```python
from build123d import *

# Parameters (mm, degrees)
SKETCH1_W               = 40
SKETCH1_H               = 60
BOSS_EXTRUDE4_DEPTH     = 2
FILLET1_R               = 5
SKETCH12_R              = 1
CUT_EXTRUDE6_DEPTH      = 12
CUT_EXTRUDE7_DEPTH      = 8
CUT_EXTRUDE7_DEPTH_BACK = 10
SKETCH13_R              = 1


with BuildPart() as part:
    # Sketch1 → Boss-Extrude4 (new body)
    with BuildSketch(Plane.XY):
        with Locations((-45.9850693, -3.193565597)):
            Rectangle(SKETCH1_W, SKETCH1_H)
    extrude(amount=-BOSS_EXTRUDE4_DEPTH)

    # Fillet1
    fillet1_edges = [part.edges().sort_by_distance(p)[0] for p in [
        (-65.9850693, 26.806434403, -1),
        (-65.9850693, -33.193565597, -1),
        (-25.9850693, -33.193565597, -1),
        (-25.9850693, 26.806434403, -1),
    ]]
    fillet(fillet1_edges, radius=FILLET1_R)

    # Sketch12 → Cut-Extrude6 (cut)
    with BuildSketch(Plane(origin=(0, 0, -2), x_dir=(-1, 0, 0), z_dir=(0, 0, -1))):
        with Locations((45.9850693, -3.193565597)):
            Circle(SKETCH12_R)
    extrude(amount=-CUT_EXTRUDE6_DEPTH, mode=Mode.SUBTRACT)

    # Sketch13 → Cut-Extrude7 (cut, two sides: drawn at the far end of the back side and taken through both)
    with BuildSketch(Plane(origin=(0, 0, -2), x_dir=(-1, 0, 0), z_dir=(0, 0, -1)).offset(-CUT_EXTRUDE7_DEPTH_BACK)):
        with Locations((55.9850693, 4.306434403)):
            Circle(SKETCH13_R)
        with Locations((55.9850693, -10.693565597)):
            Circle(SKETCH13_R)
    extrude(amount=CUT_EXTRUDE7_DEPTH + CUT_EXTRUDE7_DEPTH_BACK, mode=Mode.SUBTRACT)


solid = part.part
```
The model under review builds one solid part; all positions refer to its coordinate system, in mm. Round coordinates to 2 decimals unless told otherwise and drop trailing zeros. Loops run counter-clockwise (first coordinate to the right, second up) from the corner with the lowest first, then second, coordinate; pieces in that order, holes last. Notation, with made-up numbers: M 53,-16.75 L 68,-16.75 A27 ccw 68,14.25 Z; hole C 20,48.5 d7. An arc over 180 degrees is marked long. Put each result on its own line as item: value.
Q1. For pin 1 (1.2 mm diameter, centred on x = -45.99, y = -3.19, fed in from -Z), flat-tipped, find the tip position at first contact; note if it passes through.
Result set:
pin 1: passes through
Q2. Mouldability with a two-part tool opening along Y and no side actions: class faces 1 (the cylindrical face through (-56.939, -10.393, -0.986)), 2 (the flat face through (-25.985, -4, -1)), 3 (the cylindrical face through (-27.41, 25.3, -1.01)) as released by +Y, released by -Y, zero draft, split by the parting line, or undercut.
Result set:
face 1: undercut
face 2: zero draft
face 3: released by +Y
Q3. Consider section A-A, the plane x = -56. Give the boundary of the cut face in (y, z), then the cut area to 3 significant figures.
Result set:
outline: M -33.19,-2 L -11.69,-2 L -11.69,0 L -33.19,0 Z; M -9.69,-2 L 3.31,-2 L 3.31,0 L -9.69,0 Z; M 5.31,-2 L 26.81,-2 L 26.81,0 L 5.31,0 Z
area: 112 mm²
Q4. To check wall thickness, follow L1, parallel to Y at x = -56, z = -1.3; L2, parallel to Y at x = -46, z = -1.3; L3, parallel to X at y = -4, z = -0.35. State the ranges of each line that lie inside material, in increasing order.
Result set:
L1: y = -33.19 to -11.69, -9.69 to 3.31, 5.31 to 26.81
L2: y = -33.19 to -4.19, -2.19 to 26.81
L3: x = -65.99 to -46.58, -45.39 to -25.99
